Autodesk Inventor part; units mm, degrees
ref_plane "YZ Plane" through (0, 0, 0) normal (1, 0, 0) x (0, 1, 0)
ref_plane "XZ Plane" through (0, 0, 0) normal (0, 1, 0) x (-1, 0, 0)
ref_plane "XY Plane" through (0, 0, 0) normal (0, 0, 1) x (1, 0, 0)
sketch "スケッチ1" plane through (0, 0, 0) normal (1, 0, 0) x (0, 1, 0)
  line L0 (0, 0) -> (2.75, 0)
  line L1 (2.75, 0) -> (2.75, -25)
  line L2 (2.75, -25) -> (0, -25)
  line L3 (0, -25) -> (0, 0)
  line L4 (2.75, 0) -> (42.75, 0)
  line L5 (42.75, 0) -> (42.75, -20)
  line L6 (42.75, -20) -> (2.75, -20)
  line L7 (2.75, -20) -> (2.75, 0)
  line L8 (42.75, 0) -> (45.5, 0)
  line L9 (45.5, 0) -> (45.5, -25)
  line L10 (45.5, -25) -> (42.75, -25)
  line L11 (42.75, -25) -> (42.75, 0)
  line L12 (22.75, 0) -> (22.75, -20)
  line L13 (45.5, 0) -> (47.25, 0)
  line L14 (47.25, 0) -> (47.25, -8)
  line L15 (47.25, -8) -> (45.5, -8)
  line L16 (45.5, -8) -> (45.5, 0)
  line L17 (0, 0) -> (-1.75, 0)
  line L18 (-1.75, 0) -> (-1.75, -8)
  line L19 (-1.75, -8) -> (0, -8)
  line L20 (0, -8) -> (0, 0)
  line L21 (47.25, 0) -> (-1.75, 0)
  line L22 (-1.75, 0) -> (-1.75, -4.05)
  line L23 (-1.75, -4.05) -> (47.25, -4.05)
  line L24 (47.25, -4.05) -> (47.25, 0)
  point P0 (2.75, -20)
  point P1 (42.75, -20)
  dimension "d0" = 45.5
  dimension "d1" = 25
  dimension "d2" = 20
  dimension "d3" = 49
  dimension "d4" = 8
  dimension "d5" = 4.05
  dimension "d11" = 40
revolve "回転1" add sketch "スケッチ1" angle 360 about axis through (0, 2.75, 0) along (0, 1, 0) contours L23 L1 L2 L3 | L3 L19 L18 L23 | L23 L12 L6 L1 | L23 L5 L6 L12 | L23 L9 L10 L11 L5 | L23 L14 L15 L9
sketch "スケッチ2" plane through (0, 2.75, 0) normal (0, 1, 0) x (1, 0, 0)
  circle A0 centre (0, 0) radius 20
  line L0 (-20, 0) -> (-20, 80)
  line L1 (-20, 80) -> (-18.5, 80)
  line L2 (-18.5, 80) -> (-18.5, 7.5993)
  circle A1 centre (0, 0) radius 20
  point P0 (0, 0)
  dimension "d7" = 80
  dimension "d8" = 1.5
extrude "押し出し1" add sketch "スケッチ2" along normal blind 40 contours A0 L0 L1 L2
sketch "スケッチ4" plane through (-20, 2.75, -80) normal (-1, 0, 0) x (0, 0, 1)
  line L0 (0, 40) -> (65, 40)
  line L1 (0, 40) -> (40, 40)
  line L2 (40, 40) -> (40, 0)
  line L3 (40, 0) -> (0, 0)
  line L4 (0, 0) -> (0, 40)
  point P0 (80, -2.75)
  dimension "d12" = 40
  dimension "d13" = 40
extrude "押し出し2" add sketch "スケッチ4" along normal blind 0.25
sketch "スケッチ5" plane through (-18.5, 2.75, -16.8152) normal (1, 0, 0) x (0, 0, -1)
  line L0 (63.1848, 0) -> (63.1848, 40)
  line L1 (0, 0) -> (63.1848, 0)
  line L2 (63.1848, 40) -> (23.1848, 40)
  line L3 (23.1848, 40) -> (23.1848, 0)
  line L4 (23.1848, 0) -> (63.1848, 0)
  line L5 (63.1848, 0) -> (63.1848, 40)
  point P0 (-16.8152, -2.75)
  dimension "d16" = 40
extrude "押し出し3" add sketch "スケッチ5" along normal blind 0.25
sketch "スケッチ6" plane through (-18.25, 2.75, -16.8152) normal (1, 0, 0) x (0, 0, -1)
  line L0 (63.1848, 40) -> (63.1848, 0)
  line L1 (63.1848, 20) -> (23.1848, 20)
  line L2 (23.1848, 0) -> (23.1848, 40)
  point P0 (-16.8152, -2.75)
  point P1 (55.6848, 30)
  point P2 (55.6848, 10)
  dimension "d19" = 20
  dimension "d20" = 7.5
hole "穴1" at (-18.25, 32.75, -72.5) at (-18.25, 12.75, -72.5) direction (-1, 0, 0) diameter 4.2 end through all
equation "\"d1\" = 0.5 * SpringD"
equation "\"d3\" = SpringWidth"
properties part number "定荷重バネ49N" material "アルミニウム 6061"
Source: CAD feature listing. Evaluate the final solid. Frame: model axes, mm. A direction names the side the tool comes from. Round coordinates to 2 decimals unless told otherwise and drop trailing zeros. Write each loop counter-clockwise with the first axis right and the second up, starting at its lowest first coordinate (ties: lowest second). Pieces come first, ordered by that corner, then holes. Notation, with made-up numbers: M 7,58.5 L 29,58.5 A16 cw 29,68.5 Z; hole C -22.5,17.25 d8. An arc over 180 degrees is marked long. Answer as a JSON object with one key per item and string values. Group by question number.
(1) Section query C-C on x = 0. Output: boundary loops of the cut face in (y, z), then the cut area to 3 significant figures.
(2) Reachability of faces 4 (the cylindrical face through (-7.81, 46.36, 1.73)), 5 (the flat face through (-6, 0, 6)), 6 (the flat face through (11, 42.75, 17)), 7 (the flat face through (-18.25, 23, -60)) from +Z, -Z, +X, -X, +Y, -Y: full face, straight path, thin tool, end or side. Return the list, or none.
(3) First-contact query: pin 1 (2 mm diameter, centred on x = -11.5, z = -20, fed in from -Y); pin 2 (6 mm diameter, centred on x = -3, y = 4, fed in from +Z); pin 3 (1.5 mm diameter, centred on x = 12.5, y = 28.5, fed in from +Z). Flat tips, straight axial feed; report the tip coordinate or a pass-through.
(4) Section query A-A on y = 32.75. Output: boundary loops of the cut face in (x, z).
(5) Section query D-D on y = 23. Output: boundary loops of the cut face in (x, z).
(6) Section query B-B on z = -72.5. Output: boundary loops of the cut face in (x, y).
(7) Mould query, pull axis Y, two halves, no side actions, for faces 1 (the cylindrical face through (3.954, 23.093, 0.878)), 2 (the flat face through (-19, 2.75, -47)), 3 (the flat face through (-18.5, 22, -24)). Classes: +Y half, -Y half, draft (parallel to the pull), parting line (faces both ways), or undercut.
(8) Ray query, line 1 (Z direction, x = 0, y = 11); line 2 (Y direction, x = 16, z = 18.5). Return the intervals inside material, ascending. Write a range as [from, to].
Computed values:
{
 "1": {"outline": "M -1.75,-8 L 0,-8 L 0,-25 L 2.75,-25 L 2.75,-20 L 42.75,-20 L 42.75,-25 L 45.5,-25 L 45.5,-8 L 47.25,-8 L 47.25,-4.05 L -1.75,-4.05 Z; M -1.75,4.05 L 47.25,4.05 L 47.25,8 L 45.5,8 L 45.5,25 L 42.75,25 L 42.75,20 L 2.75,20 L 2.75,25 L 0,25 L 0,8 L -1.75,8 Z", "area": "1,530 mm^2"},
 "2": {"face 4": "+Y", "face 5": "-Y", "face 6": "none", "face 7": "-Z, +X, +Y, -Y"},
 "3": {"pin 1": "y = 0", "pin 2": "z = 25", "pin 3": "z = 16.18"},
 "4": {"outline": "M -20.25,-80 L -18.25,-80 L -18.25,-74.6 L -20.25,-74.6 Z; M -20.25,-70.4 L -18.25,-70.4 L -18.25,-40 L -18.5,-40 L -18.5,-7.6 A20 ccw long -20,0 L -20,-40 L -20.25,-40 Z; hole C 0,0 d8.1"},
 "5": {"outline": "M -20.25,-80 L -18.25,-80 L -18.25,-40 L -18.5,-40 L -18.5,-7.6 A20 ccw long -20,0 L -20,-40 L -20.25,-40 Z; hole C 0,0 d8.1"},
 "6": {"outline": "M -20.25,2.75 L -18.25,2.75 L -18.25,10.65 L -20.25,10.65 Z; M -20.25,14.85 L -18.25,14.85 L -18.25,30.65 L -20.25,30.65 Z; M -20.25,34.85 L -18.25,34.85 L -18.25,42.75 L -20.25,42.75 Z"},
 "7": {"face 1": "draft", "face 2": "-Y half", "face 3": "undercut"},
 "8": {"line 1": "[-20, -4.05], [4.05, 20]", "line 2": "[0, 2.75], [42.75, 45.5]"}
}
